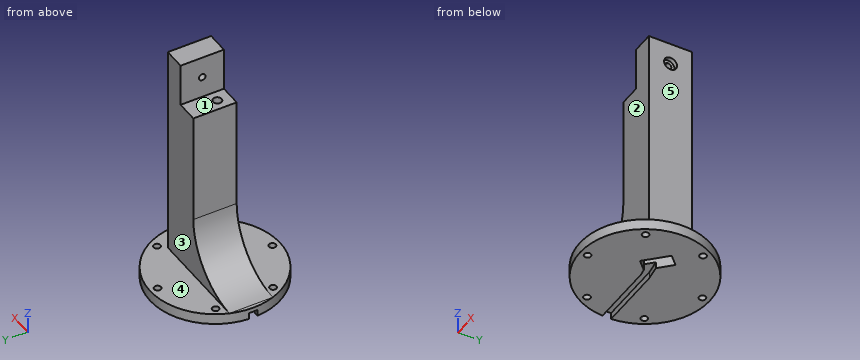
```python
from build123d import *

# Parameters (mm, degrees)
SKETCH_1_W          = 20
SKETCH_1_H          = 20
EXTRUDE_1_DEPTH     = 140
SKETCH_2_R          = 30
SKETCH_2_R_2        = 1.55
EXTRUDE_2_DEPTH     = 5
SKETCH_3_W          = 28.284271248
SKETCH_3_H          = 20
EXTRUDE_3_DEPTH     = 28.28427125
CUT_EXTRUDE_1_DEPTH = 28.28427125
CUT_EXTRUDE_2_DEPTH = 28.28427125
CUT_EXTRUDE_3_DEPTH = 28.28427125
SKETCH_8_R          = 3
CUT_EXTRUDE_4_DEPTH = 2
SKETCH_9_R          = 2
CUT_EXTRUDE_5_DEPTH = 100
CUT_EXTRUDE_6_DEPTH = 3
CUT_EXTRUDE_7_DEPTH = 3
SKETCH_12_W         = 20
SKETCH_12_H         = 20
SKETCH_12_R         = 2
EXTRUDE_5_DEPTH     = 3
CUT_EXTRUDE_START   = -35
SKETCH_13_R         = 2
CUT_EXTRUDE_8_DEPTH = 35
CUT_EXTRUDE_9_DEPTH = 3
EXTRUDE_START       = -35
EXTRUDE_6_DEPTH     = 35


with BuildPart() as part:
    # 草图1 → 凸台-拉伸1 (new body)
    with BuildSketch(Plane.XY):
        with Locations((-6.377546769, -6.820183169)):
            Rectangle(SKETCH_1_W, SKETCH_1_H)
    extrude(amount=EXTRUDE_1_DEPTH)

    # 草图2 → 凸台-拉伸2 (add)
    with BuildSketch(Plane(origin=(0, 0, 0), x_dir=(-1, 0, 0), z_dir=(0, 0, -1))):
        with Locations((16.377546769, -6.820183169)):
            Circle(SKETCH_2_R)
        with Locations((-6.572126431, 6.429816831)):
            Circle(SKETCH_2_R_2, mode=Mode.SUBTRACT)
        with Locations((16.377546769, 19.679816831)):
            Circle(SKETCH_2_R_2, mode=Mode.SUBTRACT)
        with Locations((39.32721997, 6.429816831)):
            Circle(SKETCH_2_R_2, mode=Mode.SUBTRACT)
        with Locations((39.32721997, -20.070183169)):
            Circle(SKETCH_2_R_2, mode=Mode.SUBTRACT)
        with Locations((16.377546769, -33.320183169)):
            Circle(SKETCH_2_R_2, mode=Mode.SUBTRACT)
        with Locations((-6.572126431, -20.070183169)):
            Circle(SKETCH_2_R_2, mode=Mode.SUBTRACT)
    extrude(amount=EXTRUDE_2_DEPTH)

    # 草图3 → 凸台-拉伸3 (add)
    with BuildSketch(Plane.XY):
        with Locations((-30.519682393, -6.820183169)):
            Rectangle(SKETCH_3_W, SKETCH_3_H)
    extrude(amount=EXTRUDE_3_DEPTH)

    # 草图4 → 切除-拉伸1 (cut)
    with BuildSketch(Plane(origin=(0, 3.179816831, 0), x_dir=(1, 0, 0), z_dir=(0, 1, 0))):
        with BuildLine():
            Line((-44.661818017, -3e-09), (-44.661818017, -28.28427125))
            Line((-44.661818017, -28.28427125), (-16.377546769, -28.28427125))
            ThreePointArc((-16.377546769, -28.28427125), (-24.661818017, -8.28427125), (-44.661818017, -3e-09))
        make_face()
    extrude(amount=-CUT_EXTRUDE_1_DEPTH, mode=Mode.SUBTRACT)

    # 草图6 → 切除-拉伸2 (cut)
    with BuildSketch(Plane(origin=(0, 3.179816831, 0), x_dir=(1, 0, 0), z_dir=(0, 1, 0))):
        Polygon((3.622453231, -140), (3.622453231, -100), (-6.377546769, -100), (-6.377546769, -80), (-16.377546769, -80), (-16.377546769, -100), (-16.377546769, -140), align=None)
    extrude(amount=-CUT_EXTRUDE_2_DEPTH, mode=Mode.SUBTRACT)

    # 草图7 → 切除-拉伸3 (cut)
    with BuildSketch(Plane.ZY.offset(6.377546769)):
        with BuildLine():
            ThreePointArc((91.55, -6.820183169), (90.59315932, -5.388169893), (88.903984489, -5.724167658))
            Line((88.903984489, -5.724167658), (91.096015511, -7.91619868))
            ThreePointArc((91.096015511, -7.91619868), (91.432013275, -7.413342489), (91.55, -6.820183169))
        make_face()
        with BuildLine():
            Line((91.096015511, -7.91619868), (88.903984489, -5.724167658))
            ThreePointArc((88.903984489, -5.724167658), (88.903984489, -7.91619868), (91.096015511, -7.91619868))
        make_face()
    extrude(amount=-CUT_EXTRUDE_3_DEPTH, mode=Mode.SUBTRACT)

    # 草图8 → 切除-拉伸4 (cut)
    with BuildSketch(Plane(origin=(3.622453231, 0, 0), x_dir=(0, 0, -1), z_dir=(1, 0, 0))):
        with Locations(Location((-90, -6.820183169, 0), (0, 0, 90))):
            Circle(SKETCH_8_R)
    extrude(amount=-CUT_EXTRUDE_4_DEPTH, mode=Mode.SUBTRACT)

    # 草图9 → 切除-拉伸5 (cut)
    with BuildSketch(Plane.XY.offset(80)):
        with Locations((-11.377546769, -10.820183169)):
            Circle(SKETCH_9_R)
    extrude(amount=-CUT_EXTRUDE_5_DEPTH, mode=Mode.SUBTRACT)

    # 草图10 → 切除-拉伸6 (cut)
    with BuildSketch(Plane(origin=(0, 0, -5), x_dir=(-1, 0, 0), z_dir=(0, 0, -1))):
        Polygon((11.377546769, -10.820183169), (12.756937733, -12.268495932), (16.377546769, -8.820183169), (50.683077944, -8.820183169), (50.683077944, -4.820183169), (16.377546769, -4.820183169), (10.220185265, -9.18901728), align=None)
    extrude(amount=-CUT_EXTRUDE_6_DEPTH, mode=Mode.SUBTRACT)

    # 草图11 → 切除-拉伸7 (cut)
    with BuildSketch(Plane(origin=(0, 0, -5), x_dir=(-1, 0, 0), z_dir=(0, 0, -1))):
        Polygon((-3.622453231, -6.820183169), (-3.622453231, 3.179816831), (16.377546769, 3.179816831), (16.377546769, -16.820183169), (-3.622453231, -16.820183169), align=None)
    extrude(amount=-CUT_EXTRUDE_7_DEPTH, mode=Mode.SUBTRACT)

    # 草图12 → 凸台-拉伸5 (add)
    with BuildSketch(Plane(origin=(0, 0, -2), x_dir=(-1, 0, 0), z_dir=(0, 0, -1))):
        with Locations((6.377546769, -6.820183169)):
            Rectangle(SKETCH_12_W, SKETCH_12_H)
        with Locations(Location((11.377546769, -10.820183169, 0), (0, 0, 180))):
            Circle(SKETCH_12_R, mode=Mode.SUBTRACT)
    extrude(amount=EXTRUDE_5_DEPTH)

    # 草图13 → 切除-拉伸8 (cut)
    with BuildSketch(Plane(origin=(0, 0, -5), x_dir=(-1, 0, 0), z_dir=(0, 0, -1)).offset(CUT_EXTRUDE_START)):
        with Locations(Location((11.377546769, -10.820183169, 0), (0, 0, 180))):
            Circle(SKETCH_13_R)
        Polygon((-0.339967652, -4.345309435), (3.902673035, -0.102668747), (8.498867113, -4.698862825), (13.095061191, -9.295056903), (8.852420504, -13.53769759), (4.256226426, -8.941503512), align=None)
    extrude(amount=CUT_EXTRUDE_8_DEPTH, mode=Mode.SUBTRACT)

    # 草图14 → 切除-拉伸9 (cut)
    with BuildSketch(Plane(origin=(0, 0, -5), x_dir=(-1, 0, 0), z_dir=(0, 0, -1))):
        Polygon((13.095061191, -9.295056903), (16.377546769, -8.820183169), (16.377546769, -4.820183169), (9.60060106, -5.800596772), align=None)
    extrude(amount=-CUT_EXTRUDE_9_DEPTH, mode=Mode.SUBTRACT)

    # 草图15 → 凸台-拉伸6 (add)
    with BuildSketch(Plane(origin=(0, 0, -5), x_dir=(-1, 0, 0), z_dir=(0, 0, -1)).offset(EXTRUDE_START)):
        with BuildLine():
            Line((10.062802613, -12.32731548), (12.884679081, -9.505439013))
            ThreePointArc((12.884679081, -9.505439013), (12.791760332, -12.234396731), (10.062802613, -12.32731548))
        make_face()
    extrude(amount=EXTRUDE_6_DEPTH)


solid = part.part
```
Build history of the part. All positions in model axes, mm. Face numbers are marked on the shaded views. A direction names the side the tool comes from. Round coordinates to 2 decimals unless told otherwise and drop trailing zeros. Loops run counter-clockwise (first coordinate to the right, second up) from the corner with the lowest first, then second, coordinate; pieces in that order, holes last.
Item 1: Saw through at B-B (x = -42). List the corners of the cut face in (y, z).
Item 2: Which spindle directions (+Z, -Z, +X, -X, +Y, -Y) get a long thin tool onto all of the face, cutting with end or side? Do the marked faces 1, 2, 3, 4 and 5. Say none if no direction does.
Item 3: Saw through at C-C (x = 6.5). List the corners of the cut face in (y, z), then the cut area to 3 significant figures.
Item 4: Saw through at D-D (z = 31.5). List the corners of the cut face in (x, y).
Item 5: Drill centre lines: line 1 along Y through (x, z) = (-6, 37); line 2 along Z through (x, y) = (-13.5, -14.5); line 3 along Z through (x, y) = (-29.5, 20). Where is each one in solid material? Low to high.
Item 6: Saw through at A-A (z = 90). List the corners of the cut face in (x, y), then the cut area to 3 significant figures.
Item 7: Pin check, flat tips, straight feed: P1, Ø3, axis at x = 6.57, y = 6.43, coming from the -Z side (1 decimal); P2, Ø10, axis at x = -2, z = 39.5, coming from the -Y side; P3, Ø3.5, axis at x = -29.5, z = -3, coming from the +Y side; P4, Ø5, axis at y = -6, z = 76.5, coming from the -X side. Stop position of each tip, or through.
Worked answers:
1. outline: (-22.42, -5) - (-8.82, -5) - (-8.82, -2) - (-4.82, -2) - (-4.82, -5) - (8.78, -5) - (8.78, 0) - (3.18, 0) - (3.18, 0.13) - (-16.82, 0.13) - (-16.82, 0) - (-22.42, 0) - close
2. face 1: +Z, -X, +Y, -Y
2. face 2: +Z, +X, -X, -Y
2. face 3: +Z, +X, -X, +Y
2. face 4: +Z, +X
2. face 5: +Z, +X, +Y, -Y
3. outline: (-26.23, -5) - (-21.62, -5) - (-21.62, 0) - (-26.23, 0) - close; (-18.52, -5) - (4.88, -5) - (4.88, 0) - (-18.52, 0) - close; (7.98, -5) - (12.59, -5) - (12.59, 0) - (7.98, 0) - close
3. area: 163 mm2
4. outline: (-16.38, -16.82) - (3.62, -16.82) - (3.62, 3.18) - (-16.38, 3.18) - close; hole circle Ø4 at (-11.38, -10.82)
5. line 1: y = -16.82 to 3.18
5. line 2: z = -5 to 80
5. line 3: z = -5 to 0
6. outline: (-6.38, -16.82) - (3.62, -16.82) - (3.62, -9.82) - (1.62, -9.82) - (1.62, -8.37) - (-6.38, -8.37) - close; (-6.38, -5.27) - (1.62, -5.27) - (1.62, -3.82) - (3.62, -3.82) - (3.62, 3.18) - (-6.38, 3.18) - close
6. area: 163 mm2
7. P1: passes through
7. P2: stops at y = -16.82
7. P3: stops at y = 20.94
7. P4: stops at x = -16.38
